from build123d import *

# Parameters (mm, degrees)
F0_W     = 325.12
F0_H     = 436.88
F1_DEPTH = 231.14
F2_T     = -3.175
F4_DEPTH = 436.881


with BuildPart() as f1:
    # F0 (on Top) → F1 (new body)
    with BuildSketch(Plane.XY):
        Rectangle(F0_W, F0_H)
    extrude(amount=F1_DEPTH)

    # F2
    f2_openings = [f1.faces().sort_by_distance(p)[0] for p in [
        (0, 0, 231.14),
    ]]
    offset(amount=F2_T, openings=f2_openings)

    # F3 (on face) → F4 (cut, through all)
    with BuildSketch(Plane.XZ.offset(218.44)):
        with BuildLine():
            ThreePointArc((-50.8, 193.04), (-63.5, 180.34), (-50.8, 167.64))
            Line((-50.8, 167.64), (50.8, 167.64))
            ThreePointArc((50.8, 167.64), (63.5, 180.34), (50.8, 193.04))
            Line((50.8, 193.04), (-50.8, 193.04))
        make_face()
    extrude(amount=-F4_DEPTH, mode=Mode.SUBTRACT)


solid = f1.part
Here's how the part is built. I have some questions about the finished solid (model axes, mm). A direction names the side the tool comes from. Round coordinates to 2 decimals unless told otherwise and drop trailing zeros. Write each loop counter-clockwise with the first axis right and the second up, starting at its lowest first coordinate (ties: lowest second). Pieces come first, ordered by that corner, then holes.
1. Suppose I cut it at C-C (y = -28.5). List the corners of the cut face in (x, z) for me (3 decimals).
2. For faces 1 (the cylindrical face through (63.497, -216.875, 180.061)), 2 (the flat face through (-2, -215.265, 116)), 3 (the flat face through (-2, -218.44, 114)), which set-ups out of +Z, -Z, +X, -X, +Y, -Y let a thin tool reach every point of the face, with its end or its side?
3. I need wall thicknesses on L1, parallel to X at y = -167, z = 144 (3 decimals); L2, parallel to Y at x = 31.5, z = 116 (3 decimals); L3, parallel to Z at x = 45.5, y = -31 (3 decimals). Which ranges of each line are inside material? Lowest first, please.
4. If we mould it in two halves opening along Y, with no side actions, what happens to faces 4 (the cylindrical face through (-63.497, 216.83, 180.619)), 5 (the flat face through (-2, 3, 3.175)), 6 (the flat face through (-2, 218.44, 114))? For each: released by +Y, released by -Y, zero draft, split by the parting line, or undercut.
5. Suppose I cut it at A-A (x = 0.5). List the corners of the cut face in (y, z) for me (3 decimals), and give its area (3 significant figures).
6. Suppose I cut it at B-B (z = 108.5). List the corners of the cut face in (x, y) for me (3 decimals).
7. Suppose I cut it at D-D (z = 180). List the corners of the cut face in (x, y) for me (3 decimals).
8. Will this pin go through, and if not, where does the flat tip stop? pin 1 Ø12 at (x, y) = (63.5, 59.5) entering from +Z (3 decimals).
Answer sheet:
1. outline: (-162.56, 0) - (162.56, 0) - (162.56, 231.14) - (159.385, 231.14) - (159.385, 3.175) - (-159.385, 3.175) - (-159.385, 231.14) - (-162.56, 231.14) - close
2. face 1: +Y, -Y
2. face 2: +Z
2. face 3: +Z, -Z, +X, -X, -Y
3. L1: x = -162.56 to -159.385, 159.385 to 162.56
3. L2: y = -218.44 to -215.265, 215.265 to 218.44
3. L3: z = 0 to 3.175
4. face 4: zero draft
4. face 5: undercut
4. face 6: released by +Y
5. outline: (-218.44, 0) - (218.44, 0) - (218.44, 167.64) - (215.265, 167.64) - (215.265, 3.175) - (-215.265, 3.175) - (-215.265, 167.64) - (-218.44, 167.64) - close; (-218.44, 193.04) - (-215.265, 193.04) - (-215.265, 231.14) - (-218.44, 231.14) - close; (215.265, 193.04) - (218.44, 193.04) - (218.44, 231.14) - (215.265, 231.14) - close
5. area: 2,670 mm2
6. outline: (-162.56, -218.44) - (162.56, -218.44) - (162.56, 218.44) - (-162.56, 218.44) - close; hole (-159.385, -215.265) - (159.385, -215.265) - (159.385, 215.265) - (-159.385, 215.265) - close
7. outline: (-162.56, -218.44) - (-63.495, -218.44) - (-63.495, -215.265) - (-159.385, -215.265) - (-159.385, 215.265) - (-63.495, 215.265) - (-63.495, 218.44) - (-162.56, 218.44) - close; (63.495, -218.44) - (162.56, -218.44) - (162.56, 218.44) - (63.495, 218.44) - (63.495, 215.265) - (159.385, 215.265) - (159.385, -215.265) - (63.495, -215.265) - close
8. pin 1: stops at z = 3.175
